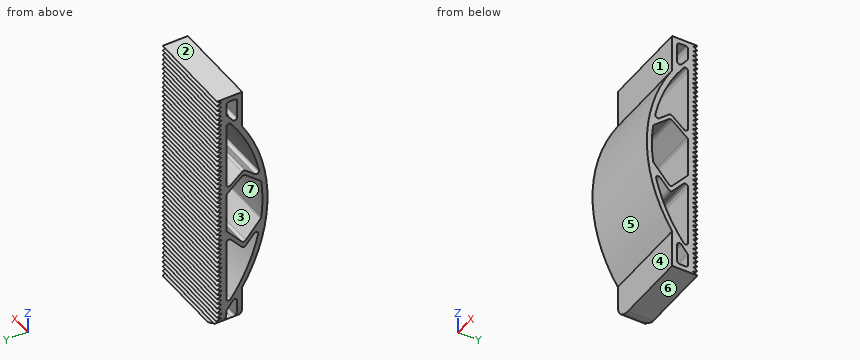
```python
from build123d import *

# Parameters (mm, degrees)
SKETCH1_W           = 35
SKETCH1_H           = 100
BOSS_EXTRUDE1_DEPTH = 10
CUT_EXTRUDE1_DEPTH  = 107.418983269
LPATTERN1_COUNT     = 50
LPATTERN1_PITCH     = 2
BOSS_EXTRUDE2_DEPTH = 35
FILLET1_R           = 6.5
SKETCH5_W           = 5.628511334
SKETCH5_H           = 4.267949192
CUT_EXTRUDE2_DEPTH  = 107.418983269
FILLET2_R           = 1


with BuildPart() as part:
    # Sketch1 → Boss-Extrude1 (new body)
    with BuildSketch(Plane(origin=(0, 0, 0), x_dir=(1, 0, 0), z_dir=(0, 1, 0))):
        with Locations((17.5, 50)):
            Rectangle(SKETCH1_W, SKETCH1_H)
    extrude(amount=BOSS_EXTRUDE1_DEPTH)

    # Sketch3 → Cut-Extrude1 (cut, through all)
    with BuildSketch(Plane.ZY):
        Polygon((-100, 10), (-99, 8.267949192), (-98, 10), align=None)
    cut_extrude1 = extrude(amount=-CUT_EXTRUDE1_DEPTH, mode=Mode.SUBTRACT)

    # LPattern1: Cut-Extrude1 ×50
    with Locations(*[(0, 0, i * LPATTERN1_PITCH) for i in range(1, LPATTERN1_COUNT)]):
        add(cut_extrude1, mode=Mode.SUBTRACT)

    # Sketch4 → Boss-Extrude2 (add)
    with BuildSketch(Plane(origin=(35, 0, 0), x_dir=(0, 0, -1), z_dir=(1, 0, 0))):
        with BuildLine():
            Line((15, 0), (85, 0))
            ThreePointArc((85, 0), (50, -10), (15, 0))
        make_face()
    extrude(amount=-BOSS_EXTRUDE2_DEPTH)

    # Fillet1
    fillet1_edges = [part.edges().sort_by_distance(p)[0] for p in [
        (0, 5, -100),
    ]]
    fillet(fillet1_edges, radius=FILLET1_R)

    # Sketch5 → Cut-Extrude2 (cut, through all)
    with BuildSketch(Plane.ZY):
        with Locations((-95.185744333, 4.133974596)):
            Rectangle(SKETCH5_W, SKETCH5_H)
        with BuildLine():
            ThreePointArc((-92.371488666, 6.267949192), (-89.617737689, 4.058206439), (-86.748958552, 2))
            Line((-86.748958552, 2), (-92.371488666, 2))
            Line((-92.371488666, 2), (-92.371488666, 6.267949192))
        make_face()
        with BuildLine():
            Line((-60.299711515, 6.267949192), (-90.371488666, 6.267949192))
            ThreePointArc((-90.371488666, 6.267949192), (-76.431686672, -2.311322045), (-60.776399584, -7.08981143))
            Line((-60.776399584, -7.08981143), (-68.299711515, -0.616025404))
            Line((-68.299711515, -0.616025404), (-60.299711515, 6.267949192))
        make_face()
        with BuildLine():
            Line((-42, 6.267949192), (-58, 6.267949192))
            Line((-58, 6.267949192), (-66, -0.616025404))
            Line((-66, -0.616025404), (-58, -7.5))
            ThreePointArc((-58, -7.5), (-50, -8), (-42, -7.5))
            Line((-42, -7.5), (-36.160154055, -0.616025404))
            Line((-36.160154055, -0.616025404), (-42, 6.267949192))
        make_face()
        with BuildLine():
            Line((-9.628511334, 6.267949192), (-40.032965827, 6.267949192))
            Line((-40.032965827, 6.267949192), (-34.193119883, -0.616025404))
            Line((-34.193119883, -0.616025404), (-39.760500511, -7.178819556))
            ThreePointArc((-39.760500511, -7.178819556), (-23.816571501, -2.422741303), (-9.628511334, 6.267949192))
        make_face()
        with Locations((-4.814255667, 4.133974596)):
            Rectangle(SKETCH5_W, SKETCH5_H)
        with BuildLine():
            Line((-7.628511334, 6.267949192), (-7.628511334, 2))
            Line((-7.628511334, 2), (-13.251041448, 2))
            ThreePointArc((-13.251041448, 2), (-10.382262311, 4.058206439), (-7.628511334, 6.267949192))
        make_face()
    extrude(amount=-CUT_EXTRUDE2_DEPTH, mode=Mode.SUBTRACT)

    # Fillet2
    fillet2_edges = [part.edges().sort_by_distance(p)[0] for p in [
        (17.5, -7.5, -58),
        (17.5, -0.616025404, -66),
        (17.5, 6.267949192, -58),
        (17.5, 6.267949192, -42),
        (17.5, -0.616025404, -36.160154055),
        (17.5, -7.5, -42),
        (17.5, 6.267949192, -90.371488666),
        (17.5, 6.267949192, -60.299711515),
        (17.5, -0.616025404, -68.299711515),
        (17.5, -7.08981143, -60.776399584),
        (17.5, 6.267949192, -7.628511334),
        (17.5, 6.267949192, -2),
        (17.5, 2, -2),
        (17.5, 2, -13.251041448),
        (17.5, -7.178819556, -39.760500511),
        (17.5, -0.616025404, -34.193119883),
        (17.5, 6.267949192, -40.032965827),
        (17.5, 6.267949192, -9.628511334),
        (17.5, 2, -86.748958552),
        (18.40479212, 2, -98),
        (18.40479212, 6.267949192, -98),
        (17.5, 6.267949192, -92.371488666),
    ]]
    fillet(fillet2_edges, radius=FILLET2_R)


solid = part.part
```
Source: CAD feature listing. Evaluate the final solid. Frame: model axes, mm. Face numbers are marked on the shaded views. A direction names the side the tool comes from. Round coordinates to 2 decimals unless told otherwise and drop trailing zeros. One line per item, written item: value. Start each with the question number.
Q1. Pin query (flat end, axial travel): pin 1 (7.5 mm diameter, centred on x = 14, z = -96, fed in from -Y); pin 2 (19.5 mm diameter, centred on x = 10, z = -71.5, fed in from -Y); pin 3 (6 mm diameter, centred on x = 15, z = -17.5, fed in from -Y). Return the tip coordinate at first contact, or that it passes through.
Q2. Section query A-A (x = 15). Give the number of separate pieces and of enclosed holes in the cut face, plus the area to 3 significant figures.
Q3. Draft query along Y for the marked faces 5, 6 and 7. Return one class per face: pulls with the +Y half, pulls with the -Y half, needs draft (parallel to the pull), parting line crosses it, or undercut.
Q4. Material intervals for probe 1 along Z at (x, y) = (19.5, 2.5); probe 2 along Z at (x, y) = (21.5, 1.5); probe 3 along Z at (x, y) = (19.5, -1.25), sorted ascending.
Q5. Access query for the marked faces 1, 2, 3 and 4. Directions: +Z, -Z, +X, -X, +Y, -Y. A direction counts if a zero-diameter tool reaches every point of the face in a straight line with its end or side. Return the directions, or none.
Findings below:
1. pin 1: y = 0
1. pin 2: y = -8.95
1. pin 3: y = -3.07
2. separate pieces: 1
2. enclosed holes: 5
2. area: 602 mm²
3. face 5: pulls with the -Y half
3. face 6: needs draft
3. face 7: undercut
4. probe 1: -100 to -97.87, -89.01 to -85.2, -64.68 to -62.38, -38.8 to -36.84, -14.8 to -10.99, -2.13 to 0
4. probe 2: -100 to -83.62, -65.84 to -63.54, -37.96 to -35.99, -16.38 to 0
4. probe 3: -82.91 to -78.67, -67.54 to -65.24, -36.7 to -34.73, -21.33 to -17.09
5. face 1: +Z, +X, -X, -Y
5. face 2: +Z, +X, -X, +Y, -Y
5. face 3: +X, -X
5. face 4: -Z, +X, -X, -Y
